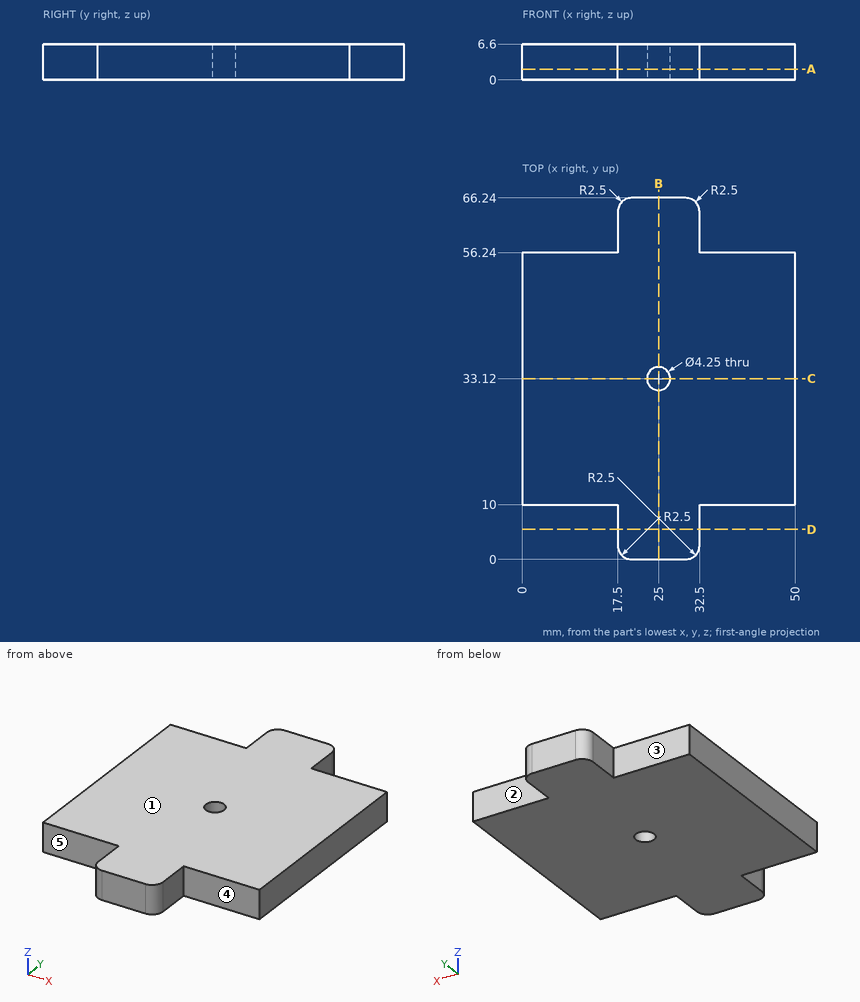
The drawing under review shows one solid part. Ordinate dimensions are in mm from its lowest x, y, z. A direction names the side the tool comes from. Round coordinates to 2 decimals unless told otherwise and drop trailing zeros. Write each loop counter-clockwise with the first axis right and the second up, starting at its lowest first coordinate (ties: lowest second). Pieces come first, ordered by that corner, then holes. Notation, with made-up numbers: M 77.25,89 L 89.25,89 A23 ccw 89.25,98 Z; hole C 13,2.5 d5. An arc over 180 degrees is marked long. One line per item, written item: value. Start each with the question number.
(1) We need section A-A (z = 2). Give the boundary of the cut face in (x, y) (3 decimals), and give its area (3 significant figures).
(2) Machinability: for the marked faces 1, 2, 3, 4 and 5, which of the approach directions +Z, -Z, +X, -X, +Y, -Y give a long, thin tool a straight path to every point of the face, cutting with its end or side? Answer none if there is none.
(3) Insertion check: pin 1 (2 mm diameter, centred on y = 7, z = 4.5, fed in from -X); pin 2 (1.5 mm diameter, centred on y = 42.5, z = 3, fed in from -X); pin 3 (2 mm diameter, centred on x = 32, z = 5, fed in from +Y); pin 4 (3.5 mm diameter, centred on x = 39.5, z = 3, fed in from +Y). Each pin has a flat end and moves straight along its axis. Give the tip position at first contact, or say it passes through.
(4) We need section B-B (x = 25). Give the boundary of the cut face in (y, z) (3 decimals), and give its area (3 significant figures).
(5) We need section D-D (y = 5.5). Give the boundary of the cut face in (x, z), and give its area (3 significant figures).
(6) Wall thickness on line 1 (Y direction, x = 25, z = 5) (3 decimals); line 2 (X direction, y = 33, z = 2); line 3 (Y direction, x = 41, z = 1.75): over which ranges is each line inside the solid? List them lowest first.
(7) We need section C-C (y = 33.12). Give the boundary of the cut face in (x, z) (3 decimals).
Result:
1. outline: M 0,10 L 17.5,10 L 17.5,2.5 A2.5 ccw 20,0 L 30,0 A2.5 ccw 32.5,2.5 L 32.5,10 L 50,10 L 50,56.24 L 32.5,56.24 L 32.5,63.74 A2.5 ccw 30,66.24 L 20,66.24 A2.5 ccw 17.5,63.74 L 17.5,56.24 L 0,56.24 Z; hole C 25,33.12 d4.25
1. area: 2,590 mm²
2. face 1: +Z, +X, -X, +Y, -Y
2. face 2: +Z, -Z, +X, +Y
2. face 3: +Z, -Z, -X, +Y
2. face 4: +Z, -Z, +X, -Y
2. face 5: +Z, -Z, -X, -Y
3. pin 1: x = 17.5
3. pin 2: x = 0
3. pin 3: y = 66.03
3. pin 4: y = 56.24
4. outline: M 0,0 L 30.995,0 L 30.995,6.6 L 0,6.6 Z; M 35.245,0 L 66.24,0 L 66.24,6.6 L 35.245,6.6 Z
4. area: 409 mm²
5. outline: M 17.5,0 L 32.5,0 L 32.5,6.6 L 17.5,6.6 Z
5. area: 99.0 mm²
6. line 1: 0 to 30.995, 35.245 to 66.24
6. line 2: 0 to 22.88, 27.12 to 50
6. line 3: 10 to 56.24
7. outline: M 0,0 L 22.875,0 L 22.875,6.6 L 0,6.6 Z; M 27.125,0 L 50,0 L 50,6.6 L 27.125,6.6 Z
